```python
from build123d import *

# Parameters (mm, degrees)
SKETCH1_W           = 16
SKETCH1_H           = 5
BOSS_EXTRUDE1_DEPTH = 5


with BuildPart() as part:
    # Sketch1 → Boss-Extrude1 (new body)
    with BuildSketch(Plane(origin=(0, 0, 0), x_dir=(1, 0, 0), z_dir=(0, 1, 0))):
        with BuildLine():
            Line((-50, 60), (50, 60))
            ThreePointArc((50, 60), (64.142135624, 54.142135624), (70, 40))
            Line((70, 40), (70, -40))
            ThreePointArc((70, -40), (64.142135624, -54.142135624), (50, -60))
            Line((50, -60), (-50, -60))
            ThreePointArc((-50, -60), (-64.142135624, -54.142135624), (-70, -40))
            Line((-70, -40), (-70, 40))
            ThreePointArc((-70, 40), (-64.142135624, 54.142135624), (-50, 60))
        make_face()
        Rectangle(SKETCH1_W, SKETCH1_H, mode=Mode.SUBTRACT)
        with Locations((-32, 0)):
            Rectangle(SKETCH1_W, SKETCH1_H, mode=Mode.SUBTRACT)
        with Locations((32, 0)):
            Rectangle(SKETCH1_W, SKETCH1_H, mode=Mode.SUBTRACT)
    extrude(amount=BOSS_EXTRUDE1_DEPTH)


solid = part.part
```
Geometry check sheet. Reference: the model listing, model coordinates, mm. A direction names the side the tool comes from. Coordinates: 2 decimals unless noted, no trailing zeros. Order: outer loops, then holes, each group sorted by start corner. A loop starts at its lowest first (then second) coordinate and runs counter-clockwise, first axis right, second up. Notation, with made-up numbers: (-36, -29) - (5, -29) arc R13 cw to (5, -7) - close; hole circle Ø3 at (18, 44.25). An arc over 180 degrees is marked (long way). Use one line per item in the form item = value.
1. Draft check along Z on faces 3 (the face through (-8, 2, 0)), 4 (the face through (1, 0, -14)), 5 (the face through (-63.986, 2.465, 54.297)). Enter one of: pulls with the +Z half, pulls with the -Z half, needs draft (parallel to the pull), parting line crosses it, or undercut.
Here are the results:
face_3 = undercut
face_4 = needs draft
face_5 = pulls with the +Z half
2. Section check C-C (z = 50). Record the boundary of the cut face in (x, y), then the cut area to 3 significant figures.
Here are the results:
outline = (-67.32, 0) - (67.32, 0) - (67.32, 5) - (-67.32, 5) - close
area = 673 mm²
3. Access from +Z, -Z, +X, -X, +Y, -Y to the whole of each face (thin tool, end or side, straight path). Record for faces 1 (the face through (-70, 2, 1)), 2 (the face through (32, 2, 2.5)).
Here are the results:
face_1 = +Z, -Z, -X, +Y, -Y
face_2 = +Y, -Y
4. Section check B-B (x = 26.5). Record the boundary of the cut face in (y, z).
Here are the results:
outline = (0, -60) - (5, -60) - (5, -2.5) - (0, -2.5) - close; (0, 2.5) - (5, 2.5) - (5, 60) - (0, 60) - close
5. Scan lines: line 1 (Z direction, x = 36.5, y = 4.15); line 2 (Z direction, x = -53.5, y = 2.95); line 3 (Z direction, x = 64, y = 1.75). Record each from-to range of solid material in increasing order.
Here are the results:
line_1 = -60 to -2.5, 2.5 to 60
line_2 = -59.69 to 59.69
line_3 = -54.28 to 54.28
6. Section check D-D (x = -57.5). Record the boundary of the cut face in (y, z).
Here are the results:
outline = (0, -58.54) - (5, -58.54) - (5, 58.54) - (0, 58.54) - close
7. Section check A-A (y = 2.25). Record the boundary of the cut face in (x, z).
Here are the results:
outline = (-70, -40) arc R20 ccw to (-50, -60) - (50, -60) arc R20 ccw to (70, -40) - (70, 40) arc R20 ccw to (50, 60) - (-50, 60) arc R20 ccw to (-70, 40) - close; hole (-40, -2.5) - (-24, -2.5) - (-24, 2.5) - (-40, 2.5) - close; hole (-8, -2.5) - (8, -2.5) - (8, 2.5) - (-8, 2.5) - close; hole (24, -2.5) - (40, -2.5) - (40, 2.5) - (24, 2.5) - close
